Verification items for the finished model (mm, model axes). Face numbers are marked on the shaded views. A direction names the side the tool comes from. Coordinates: 2 decimals unless noted, no trailing zeros. Loops run counter-clockwise (first coordinate to the right, second up) from the corner with the lowest first, then second, coordinate; pieces in that order, holes last.
Q1. Sectioned sample at A-A (x = 0). Enter the section's corners in (y, z), then the cut area to 3 significant figures.
Q2. Sectioned sample at D-D (z = 1.75). Enter the section's corners in (x, y).
Q3. Access from +Z, -Z, +X, -X, +Y, -Y to the whole of each face (thin tool, end or side, straight path). Record for the marked faces 4 and 5.
Q4. Material ranges on probe 1 along Y at (x, z) = (0, 9.25); probe 2 along X at (y, z) = (6.5, 5.5); probe 3 along Y at (x, z) = (8, 14), recorded low to high.
Q5. Go/stop test with flat-tipped pins: P1, Ø10, axis at x = 2, y = -12, coming from the -Z side; P2, Ø2, axis at y = 8.5, z = 6, coming from the -X side; P3, Ø5, axis at y = 4.5, z = 7, coming from the +X side; P4, Ø8, axis at y = 7, z = 12, coming from the +X side. Record where each tip stops, or that it passes through.
Q6. Sectioned sample at C-C (z = 9.75). Enter the section's corners in (x, y).
Q7. Mould release check, pull along Y, two halves, no side actions. Record for the marked faces 1, 2 and 3: +Y half, -Y half, draft (parallel to the pull), parting line (faces both ways), or undercut.
```python
from build123d import *

# Parameters (mm, degrees)
F0_R     = 15.24
F1_DEPTH = 15.24
F2_T     = -2.286
F3_R     = 0.508
F4_R     = 0.508


with BuildPart() as f1:
    # F0 (on Top) → F1 (new body)
    with BuildSketch(Plane.XY):
        Circle(F0_R)
    extrude(amount=F1_DEPTH)

    # F2
    f2_openings = [f1.faces().sort_by_distance(p)[0] for p in [
        (0, 0, 15.24),
    ]]
    offset(amount=F2_T, openings=f2_openings)

    # F3
    f3_edges = [f1.edges().sort_by_distance(p)[0] for p in [
        (-12.954, 0, 2.286),
    ]]
    fillet(f3_edges, radius=F3_R)

    # F4
    f4_edges = [f1.edges().sort_by_distance(p)[0] for p in [
        (-15.24, 0, 0),
    ]]
    fillet(f4_edges, radius=F4_R)


solid = f1.part
```
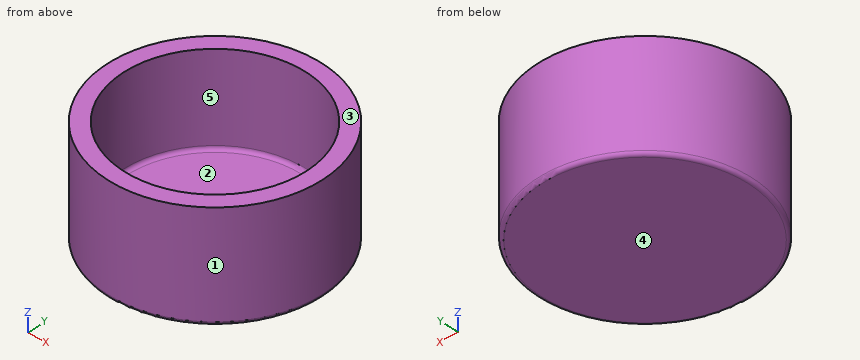
Geometry check:
1. outline: (-15.24, 0.51) arc R0.51 ccw to (-14.73, 0) - (14.73, 0) arc R0.51 ccw to (15.24, 0.51) - (15.24, 15.24) - (12.95, 15.24) - (12.95, 2.79) arc R0.51 cw to (12.45, 2.29) - (-12.45, 2.29) arc R0.51 cw to (-12.95, 2.79) - (-12.95, 15.24) - (-15.24, 15.24) - close
1. area: 129 mm2
2. outline: circle Ø30.48 at (0, 0)
3. face 4: -Z, +X, -X, +Y, -Y
3. face 5: +Z
4. probe 1: y = -15.24 to -12.95, 12.95 to 15.24
4. probe 2: x = -13.78 to -11.21, 11.21 to 13.78
4. probe 3: y = -12.97 to -10.19, 10.19 to 12.97
5. P1: stops at z = 0
5. P2: stops at x = -13.27
5. P3: stops at x = 15.11
5. P4: stops at x = 14.94
6. outline: circle Ø30.48 at (0, 0); hole circle Ø25.91 at (0, 0)
7. face 1: parting line
7. face 2: undercut
7. face 3: draft
